Check sheet for the modelled part. Datum: model origin and axes. Units: mm. A direction names the side the tool comes from. Give positions to 0.01 mm unless a question says otherwise; leave off trailing zeros. Write each loop counter-clockwise with the first axis right and the second up, starting at its lowest first coordinate (ties: lowest second). Pieces come first, ordered by that corner, then holes. Notation, with made-up numbers: M 80,-30.75 L 98,-30.75 A22 cw 98,-10.75 Z; hole C -7,28.5 d6. An arc over 180 degrees is marked long. Use CSV: the item, a comma, the result in double quotes. Start each with the question number.
1. Scan lines: line 1 (X direction, y = 4.5, z = 6); line 2 (Z direction, x = 31.5, y = 3.95); line 3 (X direction, y = 2.75, z = 6.75). Record each from-to range of solid material in increasing order.
2. Cross-section at A-A, the plane x = 31.5. Enter the section's corners in (y, z).
3. Depth check by flat-ended pin: P1, Ø3, axis at y = 9.5, z = 3, coming from the -X side; P2, Ø2.5, axis at x = -3.5, z = 6, coming from the -Y side; P3, Ø0.8, axis at x = 21, z = 3.5, coming from the -Y side; P4, Ø5, axis at x = 31.5, z = 3, coming from the +Y side. Enter the tip coordinate at first touch or a pass-through.
4. Cross-section at C-C, the plane x = -3.5. Enter the section's corners in (y, z), and give its area (3 significant figures).
5. Access from +Z, -Z, +X, -X, +Y, -Y to the whole of each face (thin tool, end or side, straight path). Record for faces 5 (the face through (17.82, 2.97, 5.92)), 6 (the face through (-2.47, 3.45, 4.65)), 7 (the face through (17.5, 10, 6)), 8 (the face through (32.9, 0, 4.6)), 9 (the face through (34, 7, 9)).
6. Mould release check, pull along Z, two halves, no side actions. Record for faces 1 (the face through (4, 7, 6)), 2 (the face through (33.16, 2.56, 5.63)), 3 (the face through (-9.5, 3.5, 6.1)), 4 (the face through (32.725, 5.313, 4.664)): +Z half, -Z half, draft (parallel to the pull), parting line (faces both ways), or undercut.
7. Cross-section at B-B, the plane z = 6. State how many separate pieces and enclosed holes the cut face has, and give its area (3 significant figures).
8. Cross-section at D-D, the plane y = 8.5. Enter the section's corners in (x, z).
Autodesk Inventor part; units mm, degrees
ref_plane "Work Plane1" through (0, 0, 6) normal (0, 0, 1) x (1, 0, 0)
ref_plane "Work Plane3" through (14, 0, 12) normal (1, 0, 0) x (0, 0, -1)
ref_plane "YZ Plane" through (0, 0, 0) normal (1, 0, 0) x (0, 1, 0)
sketch "Sketch1" plane through (0, 0, 0) normal (0, 0, 1) x (1, 0, 0)
  line L0 (0, 0) -> (28, 0)
  line L1 (28, 0) -> (28, 13)
  line L2 (28, 13) -> (0, 13)
  line L3 (0, 13) -> (0, 0)
  circle A0 centre (7, 0) radius 4
  circle A1 centre (21, 0) radius 4 construction
  line L4 (21, 0) -> (23, 0) construction
  line L5 (20.5, 0) -> (21.5, 0) construction
  line L6 (20.5, 4) -> (21.5, 4)
  line L7 (21.5, -4) -> (20.5, -4)
  arc A2 (20.5, 4) -> (20.5, -4) centre (20.5, 0) ccw
  arc A3 (21.5, -4) -> (21.5, 4) centre (21.5, 0) ccw
  point P0 (3, 0)
  point P1 (11, 0)
  point P2 (17, 0)
  point P3 (25, 0)
  point P4 (22, 0)
  point P5 (21, 0)
  point P6 (16.5, 0)
  point P7 (25.5, 0)
  dimension "d0" = 28
  dimension "d1" = 13
  dimension "d2" = 8
  dimension "d3" = 8
  dimension "d4" = 14
  dimension "d5" = 7
  dimension "d6" = 7
  dimension "d39" = 1
  dimension "d40" = 1
extrude "Extrusion1" add sketch "Sketch1" along normal blind 12 contours L3 L2 L1 L0 A3 L6 A2 A0
chamfer "Chamfer1" distance 6 angle 45 1 edges at (28, 13, 6)
sketch "Sketch2" plane through (0, 13, 12) normal (0, 1, 0) x (1, 0, 0)
  line L0 (0, 12) -> (0, 0)
  line L1 (0, 7.25) -> (11.5, 7.25)
  line L2 (11.5, 7.25) -> (11.5, 12)
  line L3 (22, 12) -> (0, 12)
  line L4 (17.5, 12) -> (17.5, 0)
  line L5 (11, 0) -> (3, 0)
  line L6 (0, 4.75) -> (11.5, 4.75)
  line L7 (11.5, 4.75) -> (11.5, 0)
  line L8 (11, 0) -> (3, 0)
  line L9 (11.5, 12) -> (17.5, 12)
  line L10 (17.5, 0) -> (11.5, 0)
  line L11 (0, 4.75) -> (0, 7.25)
  line L12 (11.5, 7.25) -> (11.5, 4.75)
  line L13 (0, 4.75) -> (11.5, 4.75)
  line L14 (11.5, 4.75) -> (11.5, 0)
  line L15 (11.5, 0) -> (0, 0)
  line L16 (0, 0) -> (0, 4.75)
  line L17 (11, 0) -> (16.5, 0)
  line L18 (11.5, 12) -> (14, 12)
  line L19 (14, 12) -> (14, 0)
  line L20 (14, 0) -> (11.5, 0)
  line L21 (11.5, 0) -> (11.5, 12)
  line L22 (0, 7.25) -> (0.5, 8)
  line L23 (0.5, 8) -> (1, 7.25)
  line L24 (2, 7.25) -> (2.5, 8)
  line L25 (2.5, 8) -> (3, 7.25)
  line L26 (4, 7.25) -> (4.5, 8)
  line L27 (4.5, 8) -> (5, 7.25)
  line L28 (6, 7.25) -> (6.5, 8)
  line L29 (6.5, 8) -> (7, 7.25)
  line L30 (8, 7.25) -> (8.5, 8)
  line L31 (8.5, 8) -> (9, 7.25)
  line L32 (0, 12) -> (0, 0)
  line L33 (0, 6) -> (11.5, 6) construction
  line L34 (0, 4.75) -> (0.5, 4)
  line L35 (0.5, 4) -> (1, 4.75)
  line L36 (2, 4.75) -> (2.5, 4)
  line L37 (2.5, 4) -> (3, 4.75)
  line L38 (4, 4.75) -> (4.5, 4)
  line L39 (4.5, 4) -> (5, 4.75)
  line L40 (6, 4.75) -> (6.5, 4)
  line L41 (6.5, 4) -> (7, 4.75)
  line L42 (8, 4.75) -> (8.5, 4)
  line L43 (8.5, 4) -> (9, 4.75)
  point P0 (17, 0)
  point P1 (3, 0)
  dimension "d12" = 6
  dimension "d13" = 2.5
  dimension "d14" = 11.5
  dimension "d41" = 2.5
  dimension "d42" = 0.75
  dimension "d43" = 1
  dimension "d46" = 2
extrude "Extrusion2" cut sketch "Sketch2" against normal blind 6
fillet "Fillet1" [suppressed]
chamfer "Chamfer2" distance 0.5 angle 45 4 edges at (3, 0, 6) (11, 0, 6) (16.5, 0, 6) (25.5, 0, 6)
ref_plane "Work Plane1" through (0, 0, 6) normal (0, 0, 1) x (1, 0, 0)
ref_plane "Work Plane3" through (14, 0, 12) normal (1, 0, 0) x (0, 0, -1)
sketch "Sketch5" plane through (28, 0, 0) normal (0, -1, 0) x (1, 0, 0)
  circle A0 centre (3.5, 6) radius 1.5
  line L0 (-28, 0) -> (-25.5, 0)
  line L1 (0, 0) -> (0, 12)
  circle A1 centre (3.5, 6) radius 3.5
  line L2 (0, 0) -> (0, 12)
  line L3 (-6, 12) -> (0, 12)
  line L4 (0, 12) -> (5.9853, 12)
  line L5 (0, 0) -> (-6, 0)
  line L6 (0, 0) -> (5.9853, 0)
  line L7 (5.9853, 0) -> (7.7426, 1.7574)
  line L8 (5.9853, 12) -> (7.7426, 10.2426)
  circle A2 centre (3.5, 6) radius 6
  line L9 (-28, 12) -> (-25.5, 12)
  line L10 (-28, 0) -> (-28, 12)
  line L11 (-25.5, 12) -> (-25.5, 0)
  line L12 (-16.5, 0) -> (-16.5, 12)
  line L13 (-16.5, 0) -> (-12, 0)
  line L14 (-16.5, 12) -> (-12, 12)
  line L15 (-2, 0) -> (0, 0)
  line L16 (-2, 12) -> (0, 12)
  line L17 (-12, 12) -> (-12, 0)
  line L18 (-2, 0) -> (-2, 12)
  point P0 (-2.5, 12)
  point P1 (-2.5, 0)
  point P2 (0, 6)
  dimension "d26" = 3
  dimension "d28" = 7
  dimension "d38" = 135
extrude "Extrusion3" add sketch "Sketch5" against normal blind 7 contours A0 | L1 A2 L6 | A1 | L1 A2 | A2 L7 L6 | L1 L4 A2 | L4 L8 A2
sketch "Sketch6" plane through (28, 7, 0) normal (0, 1, 0) x (1, 0, 0)
  arc A0 (7.7426, -10.2426) -> (7.7426, -1.7574) centre (3.5, -6) ccw
  point P0 (-28, 0)
hole "Hole1" at (31.5, 7, 6) direction (0, -1, 0) diameter 3.4 depth 8
mirror "Mirror2" about plane through (14, 0, 12) normal (1, 0, 0) of "Extrusion3", "Hole1"
chamfer "Chamfer3" distance 1.8 angle 45 1 edges at (31.5, 7, 4.3)
equation "\"d5\" = d6"
properties part number "Magnet Mount Lower"
Worked answers:
1,line 1,"x = -9.5 to -5.2, -1.8 to 29.8, 33.2 to 37.5"
1,line 2,"z = 0 to 4.3, 7.7 to 12"
1,line 3,"x = -9.45 to -5.03, -1.97 to 4.1, 9.9 to 17.6, 24.4 to 29.97, 33.03 to 37.45"
2,outline,"M 0,0 L 7,0 L 7,2.5 L 5.2,4.3 L 0,4.3 Z; M 0,7.7 L 5.2,7.7 L 7,9.5 L 7,12 L 0,12 Z"
3,P1,"stops at x = 17.5"
3,P2,"passes through"
3,P3,"stops at y = 4"
3,P4,"stops at y = 7"
4,outline,"M 0,0 L 7,0 L 7,4.3 L 0,4.3 Z; M 0,7.7 L 7,7.7 L 7,12 L 0,12 Z"
4,area,"60.2 mm^2"
5,face 5,"+Z, -Z, -Y"
5,face 6,"+Y, -Y"
5,face 7,"+Z, -Z, -X, +Y"
5,face 8,"+Z, -Z, +X, -X, -Y"
5,face 9,"+Z, -Z, +X, +Y"
6,face 1,"draft"
6,face 2,"undercut"
6,face 3,"parting line"
6,face 4,"undercut"
7,separate pieces,"3"
7,enclosed holes,"0"
7,area,"268 mm^2"
8,outline,"M 17.5,0 L 26.5,0 L 26.5,12 L 17.5,12 Z"
